from build123d import *

# Parameters (mm, degrees)
SKETCH1_W           = 60
SKETCH1_H           = 90
BOSS_EXTRUDE1_DEPTH = 15
SKETCH2_R           = 30
BOSS_EXTRUDE2_DEPTH = 25
SKETCH3_R           = 8
BOSS_EXTRUDE3_DEPTH = 15


with BuildPart() as part:
    # Sketch1 → Boss-Extrude1 (new body)
    with BuildSketch(Plane.XY):
        Rectangle(SKETCH1_W, SKETCH1_H)
    extrude(amount=BOSS_EXTRUDE1_DEPTH)

    # Sketch2 → Boss-Extrude2 (add)
    with BuildSketch(Plane.XY.offset(15)):
        Circle(SKETCH2_R)
        with BuildLine():
            ThreePointArc((4, -14.456832295), (0, 15), (-4, -14.456832295))
            ThreePointArc((-4, -14.456832295), (0, -15), (4, -14.456832295))
        make_face(mode=Mode.SUBTRACT)
    extrude(amount=BOSS_EXTRUDE2_DEPTH)

    # Sketch3 → Boss-Extrude3 (add)
    with BuildSketch(Plane(origin=(0, 45, 0), x_dir=(1, 0, 0), z_dir=(0, 1, 0))):
        with BuildLine():
            Line((30, 0), (22.03289839, 26.599347585))
            ThreePointArc((22.03289839, 26.599347585), (0, 43), (-22.03289839, 26.599347585))
            Line((-22.03289839, 26.599347585), (-30, 0))
            Line((-30, 0), (30, 0))
        make_face()
        with Locations(Location((0, 20, 0), (0, 0, 180))):
            Circle(SKETCH3_R, mode=Mode.SUBTRACT)
    boss_extrude3 = extrude(amount=-BOSS_EXTRUDE3_DEPTH)

    # Mirror1: Boss-Extrude3 across plane
    add(boss_extrude3.mirror(Plane.ZX))


solid = part.part
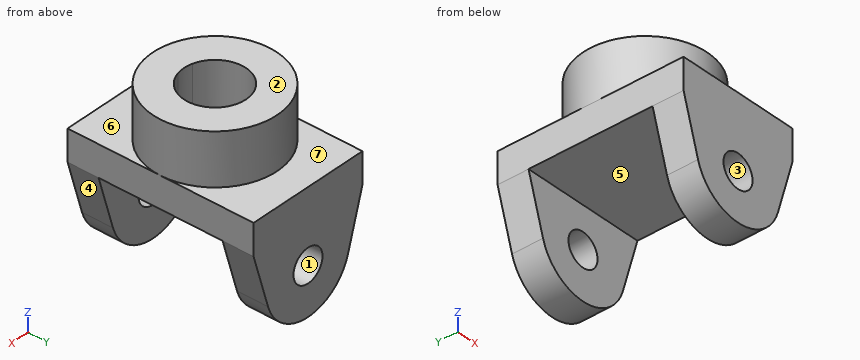
The listing builds one solid part. Answer for the finished solid, in the listing's coordinates (mm). Face numbers are marked on the shaded views. A direction names the side the tool comes from. Round coordinates to 2 decimals unless told otherwise and drop trailing zeros. Order: outer loops, then holes, each group sorted by start corner. A loop starts at its lowest first (then second) coordinate and runs counter-clockwise, first axis right, second up. Notation, with made-up numbers: (-8.5, 2.25) -> (13.5, 2.25) arc R9 ccw to (13.5, 14.25) -> close; hole circle Ø4 at (-25, 4.5). An arc over 180 degrees is marked (long way). Write each question's results on one line, items separated by ' | '. Start each with the question number.
Q1. Each of these flat-tipped pins is pushed along its axis until it touches: pin 1 (9 mm diameter, centred on x = 0, y = 1.5, fed in from +Z); pin 2 (10 mm diameter, centred on x = 4, y = -19.5, fed in from -Z); pin 3 (2 mm diameter, centred on x = -14.5, z = 21.5, fed in from +Y); pin 4 (14.5 mm diameter, centred on x = 0, z = -20, fed in from -Y). Where does it stop, or does it pass through?
Q2. Find section C-C (y = -24). Determine the outline of the cut face in (x, z), then the cut area to 3 significant figures.
Q3. The mould has two halves that part along X. Classify the marked faces 1, 2, 3 and 4: pulls with the +X half, pulls with the -X half, needs draft (parallel to the pull), parting line crosses it, or undercut.
Q4. Straight lines are drawn through the part: probe 1 along Y at (x, z) = (13.5, -5.5); probe 2 along X at (y, z) = (0.5, 27.5); probe 3 along Z at (x, y) = (22, -21). For each, find the intervals that lie inside material, in ascending order. Write a range as from..to.
Q5. Find section A-A (x = 0). Determine the outline of the cut face in (y, z), then the cut area to 3 significant figures.
Q6. Find section D-D (x = 24). Determine the outline of the cut face in (y, z), then the cut area to 3 significant figures.
Q7. Find section B-B (z = -20). Determine the outline of the cut face in (x, y), then the cut area to 3 significant figures.
Q8. Which of the six approach directions +Z, -Z, +X, -X, +Y, -Y give full straight-line access (tool end or side, diameter ignored) to the marked faces 5, 6 and 7?
Worked answers:
1) pin 1: stops at z = 15 | pin 2: stops at z = 0 | pin 3: stops at y = 26.79 | pin 4: passes through
2) outline: (-30, 0) -> (30, 0) -> (30, 15) -> (18, 15) -> (18, 40) -> (-18, 40) -> (-18, 15) -> (-30, 15) -> close | area: 1,800 mm2
3) face 1: undercut | face 2: needs draft | face 3: undercut | face 4: pulls with the +X half
4) probe 1: y = -45..-30, 30..45 | probe 2: x = -30..-14.99, 14.99..30 | probe 3: z = 0..15
5) outline: (-45, -43) -> (-30, -43) -> (-30, -28) -> (-45, -28) -> close; (-45, -12) -> (-30, -12) -> (-30, 0) -> (30, 0) -> (30, -12) -> (45, -12) -> (45, 15) -> (30, 15) -> (30, 40) -> (15, 40) -> (15, 15) -> (-15, 15) -> (-15, 40) -> (-30, 40) -> (-30, 15) -> (-45, 15) -> close; (30, -43) -> (45, -43) -> (45, -28) -> (30, -28) -> close | area: 2,910 mm2
6) outline: (-45, -20.03) -> (-30, -20.03) -> (-30, 0) -> (30, 0) -> (30, -20.03) -> (45, -20.03) -> (45, 15) -> (18, 15) -> (18, 40) -> (-18, 40) -> (-18, 15) -> (-45, 15) -> close | area: 2,850 mm2
7) outline: (-24.01, -45) -> (-8, -45) -> (-8, -30) -> (-24.01, -30) -> close; (-24.01, 30) -> (-8, 30) -> (-8, 45) -> (-24.01, 45) -> close; (8, -45) -> (24.01, -45) -> (24.01, -30) -> (8, -30) -> close; (8, 30) -> (24.01, 30) -> (24.01, 45) -> (8, 45) -> close | area: 961 mm2
8) face 5: -Z, +X, -X | face 6: +Z, -Y | face 7: +Z, +Y
